Input: part model. Units: mm. Frame: model coordinates. Face numbers are marked on the shaded views. A direction names the side the tool comes from. Give positions to 0.01 mm unless a question says otherwise; leave off trailing zeros. Write each loop counter-clockwise with the first axis right and the second up, starting at its lowest first coordinate (ties: lowest second). Pieces come first, ordered by that corner, then holes.
```python
from build123d import *

# Parameters (mm, degrees)
F3_D     = 12.7
F3_DEPTH = 101.6
F3_TIP   = 3.8154649308


with BuildPart() as f1:
    # F0 (on Front) → F1 (revolve)
    with BuildSketch(Plane.XZ):
        Polygon((14.8333879188, 76.4790847898), (0, 76.4899104834), (0, 43.3194376528), (61.6134181619, 43.3194376528), (61.6134181619, -63.8560429215), (0, -63.8560429215), (0, -76.4899104834), (76.2181654572, -76.4899104834), (76.2181654572, 56.0453906655), (14.8333879188, 56.0453906655), align=None)
    revolve(axis=Axis((0, 0, 0), (0, 0, -1)))

    # F3 (one way)
    with BuildSketch(Plane(origin=(0, 0, 56.0453906655), x_dir=(1, 0, 0), z_dir=(0, 0, -1))):
        with Locations((0, 0)):
            Circle(F3_D / 2)
    extrude(amount=-F3_DEPTH, mode=Mode.SUBTRACT)
    with Locations(Plane(origin=(0, 0, 56.0453906655), x_dir=(1, 0, 0), z_dir=(0, 0, -1))):
        with Locations((0, 0)):
            with Locations((0, 0, -(F3_DEPTH + F3_TIP / 2))):  # 118° drill point
                Cone(0, F3_D / 2, F3_TIP, mode=Mode.SUBTRACT)


solid = f1.part
```
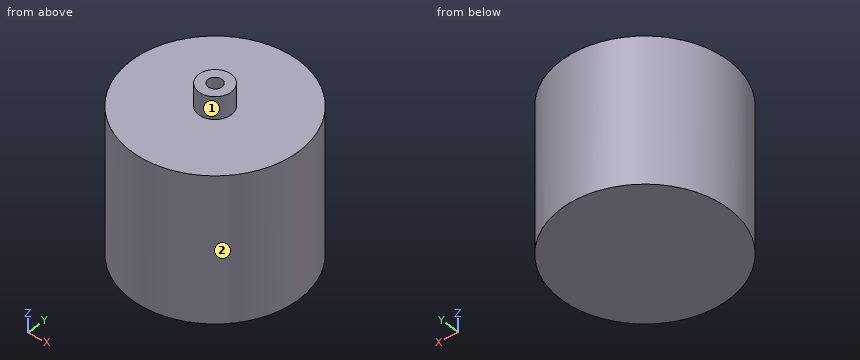
Item 1: Section D-D (y = 34). Return loops of the section in (x, z), and give its area (3 significant figures).
Item 2: Ray query, line 1 (X direction, y = 0, z = -6); line 2 (Z direction, x = -8.5, y = -20.5); line 3 (X direction, y = 0, z = 61). Return the intervals inside material, ascending.
Item 3: Section B-B (x = -46). Return loops of the section in (y, z), and give its area (3 significant figures).
Item 4: Section A-A (y = 0). Return loops of the section in (x, z), and give its area (3 significant figures).
Item 5: Pin query (flat end, axial travel): pin 1 (3 mm diameter, centred on x = 5.5, z = 19, fed in from +Y); pin 2 (3 mm diameter, centred on x = -39, z = 43.5, fed in from +Y); pin 3 (4 mm diameter, centred on x = -11, z = 35.5, fed in from +Y); pin 4 (14 mm diameter, centred on x = -1.5, y = 2, fed in from +Z). Return the tip coordinate at first contact, or that it passes through.
Item 6: Section C-C (z = -33). Return loops of the section in (x, y), and give its area (3 significant figures).
Item 7: Set-up query: the marked faces 1 and 2. Return all of +Z, -Z, +X, -X, +Y, -Y with unobstructed straight access to the full face (end or side cutting, diameter ignored); none if empty.
Solved:
1. outline: (-68.21, -76.49) - (68.21, -76.49) - (68.21, 56.05) - (-68.21, 56.05) - close; hole (-51.38, -63.86) - (51.38, -63.86) - (51.38, 43.32) - (-51.38, 43.32) - close
1. area: 7,070 mm2
2. line 1: x = -76.22 to -61.61, 61.61 to 76.22
2. line 2: z = -76.49 to -63.86, 43.32 to 56.05
2. line 3: x = -14.83 to -6.35, 6.35 to 14.83
3. outline: (-60.77, -76.49) - (60.77, -76.49) - (60.77, 56.05) - (-60.77, 56.05) - close; hole (-40.99, -63.86) - (40.99, -63.86) - (40.99, 43.32) - (-40.99, 43.32) - close
3. area: 7,320 mm2
4. outline: (-76.22, -76.49) - (76.22, -76.49) - (76.22, 56.05) - (14.83, 56.05) - (14.83, 76.48) - (6.35, 76.49) - (6.35, 56.05) - (-6.35, 56.05) - (-6.35, 76.49) - (-14.83, 76.48) - (-14.83, 56.05) - (-76.22, 56.05) - close; hole (-61.61, -63.86) - (61.61, -63.86) - (61.61, 43.32) - (-61.61, 43.32) - close
4. area: 7,340 mm2
5. pin 1: stops at y = 76.11
5. pin 2: stops at y = 66.35
5. pin 3: stops at y = 75.68
5. pin 4: stops at z = 76.49
6. outline: circle Ø152.44 at (0, 0); hole circle Ø123.23 at (0, 0)
6. area: 6,320 mm2
7. face 1: +Z
7. face 2: +Z, -Z
